Build history of the part. All positions in model axes, mm. Give positions to 0.01 mm unless a question says otherwise; leave off trailing zeros. Order: outer loops, then holes, each group sorted by start corner. A loop starts at its lowest first (then second) coordinate and runs counter-clockwise, first axis right, second up. Notation, with made-up numbers: (-9.5, -28.5) - (-5.5, -28.5) arc R7 ccw to (-5.5, -21.5) - close; hole circle Ø11 at (-28.5, 40). An arc over 180 degrees is marked (long way). Answer in a Markdown table with one row per item.
```python
from build123d import *

# Parameters (mm, degrees)
F0_W     = 146.4
F0_H     = 29.5
F1_DEPTH = 2
F2_D     = 4.4
F3_D     = 3.3
F4_D     = 8
F5_D     = 12


with BuildPart() as f1:
    # F0 (on Front) → F1 (new body)
    with BuildSketch(Plane.XZ):
        with BuildLine():
            Line((114.5, 12.8908843005), (-114.5, 12.8908843005))
            ThreePointArc((-114.5, 12.8908843005), (-114.8535533906, 12.7444376911), (-115, 12.3908843005))
            Line((-115, 12.3908843005), (-115, -66.6091156995))
            ThreePointArc((-115, -66.6091156995), (-114.8535533906, -66.9626690901), (-114.5, -67.1091156995))
            Line((-114.5, -67.1091156995), (114.5, -67.1091156995))
            ThreePointArc((114.5, -67.1091156995), (114.8535533906, -66.9626690901), (115, -66.6091156995))
            Line((115, -66.6091156995), (115, 12.3908843005))
            ThreePointArc((115, 12.3908843005), (114.8535533906, 12.7444376911), (114.5, 12.8908843005))
        make_face()
        with Locations((15.5, -19.3591156995)):
            Rectangle(F0_W, F0_H, mode=Mode.SUBTRACT)
    extrude(amount=-F1_DEPTH)

    # F2 (through all)
    with Locations(Plane.XZ):
        with Locations((-109.75, 5.3908843005), (109.75, 5.3908843005), (109.75, -59.6091156995), (-109.75, -59.6091156995)):
            Hole(F2_D / 2)

    # F3 (through all)
    with Locations(Plane.XZ):
        with Locations((-62.7, -19.3591156995), (93.7, -19.3591156995)):
            Hole(F3_D / 2)

    # F4 (through all)
    with Locations(Plane.XZ):
        with Locations((-95, -19.3591156995)):
            Hole(F4_D / 2)

    # F5 (through all)
    with Locations(Plane.XZ):
        with Locations((-50.2, -50.6091156995), (-6.4, -50.6091156995), (37.4, -50.6091156995), (81.2, -50.6091156995)):
            Hole(F5_D / 2)


solid = f1.part
```
1. Cut at D-D on z = -47. Write the cut outline in (x, y), and give its area (3 significant figures).
Check result:
| item | result |
|---|---|
| outline | (-115, 0) - (-54.99, 0) - (-54.99, 2) - (-115, 2) - close; (-45.41, 0) - (-11.19, 0) - (-11.19, 2) - (-45.41, 2) - close; (-1.61, 0) - (32.61, 0) - (32.61, 2) - (-1.61, 2) - close; (42.19, 0) - (76.41, 0) - (76.41, 2) - (42.19, 2) - close; (85.99, 0) - (115, 0) - (115, 2) - (85.99, 2) - close |
| area | 383 mm² |
2. Probe line 1 (Z direction, x = 37.4, y = 1.05); line 2 (X direction, y = 0.95, z = -50.5); line 3 (X direction, y = 1.5, z = -25). List the from-to ranges inside material, lowest first.
Check result:
| item | result |
|---|---|
| line 1 | z = -67.11 to -56.61, -44.61 to -34.11, -4.61 to 12.89 |
| line 2 | x = -115 to -56.2, -44.2 to -12.4, -0.4 to 31.4, 43.4 to 75.2, 87.2 to 115 |
| line 3 | x = -115 to -57.7, 88.7 to 115 |
3. Cut at B-B on x = 48. Write the cut outline in (y, z), and give its area (3 significant figures).
Check result:
| item | result |
|---|---|
| outline | (0, -67.11) - (2, -67.11) - (2, -34.11) - (0, -34.11) - close; (0, -4.61) - (2, -4.61) - (2, 12.89) - (0, 12.89) - close |
| area | 101 mm² |
4. Cut at C-C on x = -109.75. Write the cut outline in (y, z).
Check result:
| item | result |
|---|---|
| outline | (0, -67.11) - (2, -67.11) - (2, -61.81) - (0, -61.81) - close; (0, -57.41) - (2, -57.41) - (2, 3.19) - (0, 3.19) - close; (0, 7.59) - (2, 7.59) - (2, 12.89) - (0, 12.89) - close |
5. Cut at A-A on z = -28. Write the cut outline in (x, y), and give its area (3 significant figures).
Check result:
| item | result |
|---|---|
| outline | (-115, 0) - (-57.7, 0) - (-57.7, 2) - (-115, 2) - close; (88.7, 0) - (115, 0) - (115, 2) - (88.7, 2) - close |
| area | 167 mm² |
6. Two-plate mould, pull along X, no slides. Class faces 1 (the face through (85.62, 1.01, -46.55)), 2 (the face through (-2, 0, -35)), 3 (the face through (-98.695, 1.014, -20.891)): +X half, -X half, draft (parallel to the pull), parting line (faces both ways), or undercut.
Check result:
| item | result |
|---|---|
| face 1 | undercut |
| face 2 | draft |
| face 3 | undercut |
